```python
from build123d import *

# Parameters (mm, degrees)
DODANIE_WYCI_GNI_CIE1_DEPTH     = 58
SFAZOWANIE1_SIZE                = 10
SZKIC2_W                        = 4
SZKIC2_H                        = 58
SZKIC2_W_2                      = 3
DODANIE_WYCI_GNI_CIE2_DEPTH     = 10
SZKIC3_R                        = 2.1
SZKIC3_R_2                      = 3.1
WYTNIJ_WYCI_GNI_CIE1_DEPTH      = 108.622488356
SZKIC4_R                        = 2.1
WYTNIJ_WYCI_GNI_CIE2_DEPTH      = 101.943746711
WYTNIJ_WYCI_GNI_CIE3_DEPTH      = 168.894848045
WYTNIJ_WYCI_GNI_CIE3_DEPTH_BACK = 168.894848045
SZKIC5_W                        = 90.111418636
SZKIC5_H                        = 70.976902515


with BuildPart() as part:
    # Szkic1 → Dodanie-wyciągnięcie1 (new body)
    with BuildSketch(Plane.XY):
        Polygon((0, 0), (-4, 0), (-4, 15), (-7.2, 15), (-7.2, 0), (-10.2, 0), (-10.2, 15), (-38.4, 15), (-48.4, 25), (-48.4, 41.8), (-74.4, 41.8), (-74.4, 44.8), (-48.4, 44.8), (-48.4, 48), (-74.4, 48), (-74.4, 52), (-34.4, 52), (-34.4, 28), (0, 28), align=None)
    extrude(amount=DODANIE_WYCI_GNI_CIE1_DEPTH)

    # Sfazowanie1
    sfazowanie1_edges = [part.edges().sort_by_distance(p)[0] for p in [
        (-10.2, 15, 29),
        (-48.4, 41.8, 29),
        (-34.4, 52, 29),
        (0, 28, 29),
    ]]
    chamfer(sfazowanie1_edges, length=SFAZOWANIE1_SIZE)

    # Szkic2 → Dodanie-wyciągnięcie2 (add)
    with BuildSketch(Plane.XZ):
        with Locations((-2, 29)):
            Rectangle(SZKIC2_W, SZKIC2_H)
        with Locations((-8.7, 29)):
            Rectangle(SZKIC2_W_2, SZKIC2_H)
    extrude(amount=DODANIE_WYCI_GNI_CIE2_DEPTH)

    # Szkic3 → Wytnij-wyciągnięcie1 (cut, through all)
    with BuildSketch(Plane.XZ.offset(-41.8)):
        with Locations((-66.4, 10)):
            Circle(SZKIC3_R)
        with Locations((-66.4, 50)):
            Circle(SZKIC3_R_2)
    extrude(amount=-WYTNIJ_WYCI_GNI_CIE1_DEPTH, mode=Mode.SUBTRACT)

    # Szkic4 → Wytnij-wyciągnięcie2 (cut, through all)
    with BuildSketch(Plane.ZY.offset(10.2)):
        with Locations((14, -3)):
            Circle(SZKIC4_R)
    extrude(amount=-WYTNIJ_WYCI_GNI_CIE2_DEPTH, mode=Mode.SUBTRACT)


with BuildPart() as body_2:
    # Lustro1: mirrored copy
    add(part.part.mirror(Plane(origin=(-74.4, 52, 58), x_dir=(0, 0, 1), z_dir=(1, 0, 0))))


with BuildPart() as part_1:
    add(part.part)

    # Szkic5 → Wytnij-wyciągnięcie3 (cut, two sides: drawn at the far end of the back side and taken through both)
    with BuildSketch(Plane.XZ.offset(-41.8).offset(-WYTNIJ_WYCI_GNI_CIE3_DEPTH_BACK)):
        with Locations((-29.344290682, 35.488451258)):
            Rectangle(SZKIC5_W, SZKIC5_H)
    extrude(amount=WYTNIJ_WYCI_GNI_CIE3_DEPTH + WYTNIJ_WYCI_GNI_CIE3_DEPTH_BACK, mode=Mode.SUBTRACT)


solid = body_2.part
```
Work out the finished part from the listing and answer in its coordinate system (mm). A direction names the side the tool comes from. Round coordinates to 2 decimals unless told otherwise and drop trailing zeros. Loops run counter-clockwise (first coordinate to the right, second up) from the corner with the lowest first, then second, coordinate; pieces in that order, holes last. Notation, with made-up numbers: M -35,-37.5 L 0,-37.5 A18 ccw 0,-29.5 Z; hole C 22.5,1 d11. An arc over 180 degrees is marked long. Use CSV: the item, a comma, the result in double quotes.
Q1. Section B-B, the plane x = -92 is taken. Determine the outline of the cut face in (y, z), then the cut area to 3 significant figures.
Determined:
outline,"M 40.2,0 L 44.8,0 L 44.8,58 L 40.2,58 Z; M 48,0 L 52,0 L 52,58 L 48,58 Z"
area,"499 mm2"
Q2. Section D-D, the plane y = 7 is taken. Determine the outline of the cut face in (x, z).
Determined:
outline,"M -148.8,0 L -144.8,0 L -144.8,58 L -148.8,58 Z; M -141.6,0 L -136.6,0 L -136.6,58 L -141.6,58 Z"
Q3. Consider L1, parallel to Z at x = -82.4, y = 43.25; L2, parallel to X at y = 0, z = 3; L3, parallel to Y at x = -84.5, z = 11. Determine where each line is inside the solid, lowest interval first.
Determined:
L1,"0 to 7.9, 12.1 to 46.9, 53.1 to 58"
L2,"-148.8 to -144.8, -141.6 to -138.6"
L3,"41.8 to 44.8, 48 to 52"
Q4. Section C-C, the plane z = 50 is taken. State how many separate pieces and enclosed holes the cut face has, then the cut area to 3 significant figures.
Determined:
separate pieces,"3"
enclosed holes,"0"
area,"1,230 mm2"
Q5. The mould has two halves that part along X. Classify faces 1 (the flat face through (-83, 41.8, 29)), 2 (the flat face through (-143, 15, 29)), 3 (the flat face through (-109.5, 46.9, 28.6)): pulls with the +X half, pulls with the -X half, needs draft (parallel to the pull), parting line crosses it, or undercut.
Determined:
face 1,"needs draft"
face 2,"undercut"
face 3,"pulls with the -X half"
Q6. Each of these flat-tipped pins is pushed along its axis until it touches: pin 1 (1 mm diameter, centred on x = -144, z = 35.5, fed in from -Y); pin 2 (11 mm diameter, centred on y = 37, z = 23, fed in from -X); pin 3 (2 mm diameter, centred on x = -117, z = 47, fed in from +Y). Where does it stop, or does it pass through?
Determined:
pin 1,"y = 15"
pin 2,"x = -114.4"
pin 3,"y = 28"
Q7. Section A-A, the plane y = -3 is taken. Determine the outline of the cut face in (x, z), then the cut area to 3 significant figures.
Determined:
outline,"M -148.8,0 L -144.8,0 L -144.8,11.9 L -148.8,11.9 Z; M -148.8,16.1 L -144.8,16.1 L -144.8,58 L -148.8,58 Z; M -141.6,0 L -138.6,0 L -138.6,11.9 L -141.6,11.9 Z; M -141.6,16.1 L -138.6,16.1 L -138.6,58 L -141.6,58 Z"
area,"377 mm2"
Q8. A tool of negligible diameter and unlimited length cuts with its end or side. For faces 4 (the flat face through (-141.6, 3, 29)), 5 (the flat face through (-126, 28, 29)), 6 (the flat face through (-120, 15, 29)), 7 (the flat face through (-147, -10, 29)), 8 (the flat face through (-88, 48, 29)), from which of +Z, -Z, +X, -X, +Y, -Y can it reach the whole face along a straight path? Write none if from no direction.
Determined:
face 4,"+Z, -Z, -Y"
face 5,"+Z, -Z, -X, +Y"
face 6,"+Z, -Z, +X, -Y"
face 7,"+Z, -Z, +X, -X, -Y"
face 8,"+Z, -Z, +X"
